Geometry: see drawing. Coordinates: mm, zero at the bounding-box minimum. Coordinates: 2 decimals unless noted, no trailing zeros. Write each loop counter-clockwise with the first axis right and the second up, starting at its lowest first coordinate (ties: lowest second). Pieces come first, ordered by that corner, then holes. Notation, with made-up numbers: (56.5, -15) - (83.5, -15) arc R19 cw to (83.5, 9) - close; hole circle Ø3 at (42, 71.25). An arc over 180 degrees is marked (long way). One line per question, with ' | ' between items. Start each with the question number.
1) Section query A-A on x = 309.5. Return loops of the section in (y, z).
2) Line query: line 1 (Y direction, x = 572, z = 9.5); line 2 (X direction, y = 69, z = 13.5); line 3 (X direction, y = 25.5, z = 19). Output: solid intervals per line, ascending.
3) First-contact query: P1, Ø1.5, axis at y = 38.5, z = 16, coming from the -X side; P2, Ø10, axis at x = 203, z = 14.5, coming from the +Y side; P3, Ø4, axis at x = 496, y = 15, coming from the +Z side; P4, Ø2, axis at y = 91.5, z = 5.5, coming from the -X side. Flat tips, straight axial feed; report the tip coordinate or a pass-through.
4) Section query B-B on y = 54.5. Return loops of the section in (x, z), and give its area (3 significant figures).
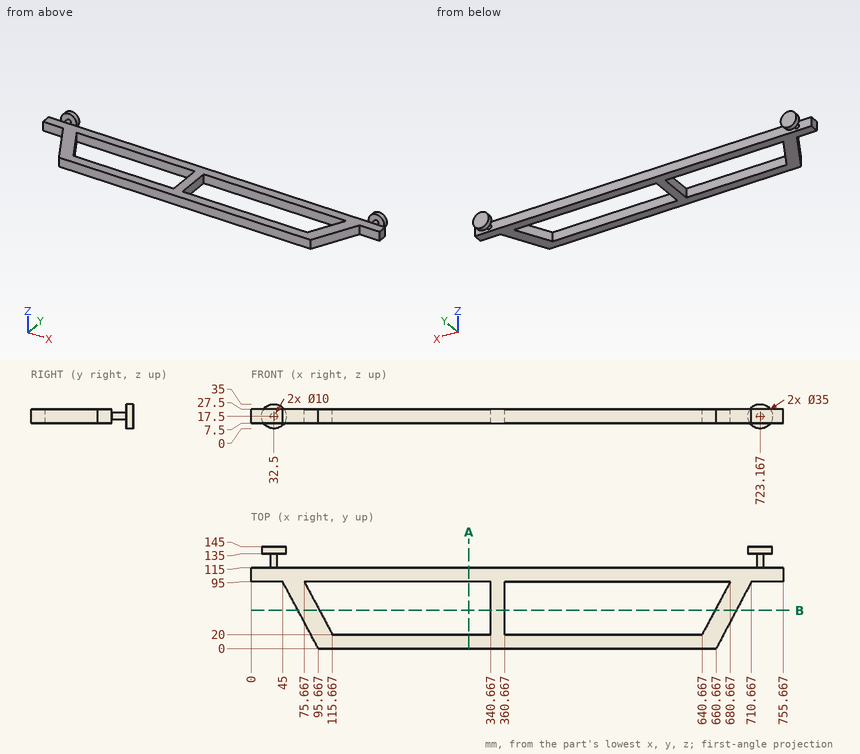
Answer key:
1) outline: (0, 7.5) - (20, 7.5) - (20, 27.5) - (0, 27.5) - close; (95, 7.5) - (115, 7.5) - (115, 27.5) - (95, 27.5) - close
2) line 1: 0 to 20, 95 to 115 | line 2: 58.87 to 89.53, 340.67 to 360.67, 666.8 to 696.98 | line 3: 82.07 to 112.73, 340.67 to 360.67, 643.6 to 674.09
3) P1: x = 74.73 | P2: y = 115 | P3: z = 27.5 | P4: through
4) outline: (66.6, 7.5) - (97.27, 7.5) - (97.27, 27.5) - (66.6, 27.5) - close; (340.67, 7.5) - (360.67, 7.5) - (360.67, 27.5) - (340.67, 27.5) - close; (659.07, 7.5) - (689.35, 7.5) - (689.35, 27.5) - (659.07, 27.5) - close | area: 1,620 mm²
